Can you work these out from the model? Positions are in its coordinate system, mm. Round coordinates to 2 decimals unless told otherwise and drop trailing zeros. Loops run counter-clockwise (first coordinate to the right, second up) from the corner with the lowest first, then second, coordinate; pieces in that order, holes last. Notation, with made-up numbers: (-27, 62) -> (15, 62) arc R21 ccw to (15, 86) -> close; hole circle Ø7 at (-21.5, 40.25). An arc over 180 degrees is marked (long way). Write each question's results on one line, items separated by ' | '.
from build123d import *

# Parameters (mm, degrees)
SKETCH_1_R          = 27
SKETCH_1_R_2        = 2
EXTRUDE_1_DEPTH     = 5
CUT_EXTRUDE_1_DEPTH = 5
SKETCH_3_R          = 1.6
CUT_EXTRUDE_2_DEPTH = 10


with BuildPart() as part:
    # 草图1 → 凸台-拉伸1 (new body)
    with BuildSketch(Plane(origin=(0, 0, 0), x_dir=(1, 0, 0), z_dir=(0, 1, 0))):
        with Locations(Location((0, 0, 0), (0, 0, 270))):
            Circle(SKETCH_1_R)
        with Locations(Location((0, 0, 0), (0, 0, 270))):
            Circle(SKETCH_1_R_2, mode=Mode.SUBTRACT)
    extrude(amount=EXTRUDE_1_DEPTH)

    # 草图2 → 切除-拉伸1 (cut)
    with BuildSketch(Plane(origin=(0, 5, 0), x_dir=(1, 0, 0), z_dir=(0, 1, 0))):
        Polygon((-3.492969129, -6.05), (3.492969129, -6.05), (6.985938257, 0), (3.492969129, 6.05), (-3.492969129, 6.05), (-6.985938257, 0), align=None)
    extrude(amount=-CUT_EXTRUDE_1_DEPTH, mode=Mode.SUBTRACT)

    # 草图3 → 切除-拉伸2 (cut)
    with BuildSketch(Plane(origin=(0, 5, 0), x_dir=(1, 0, 0), z_dir=(0, 1, 0))):
        with Locations(Location((0, 25, 0), (0, 0, 270))):
            Circle(SKETCH_3_R)
        with Locations(Location((8.550503583, 23.49231552, 0), (0, 0, 270))):
            Circle(SKETCH_3_R)
        with Locations(Location((16.069690242, 19.151111078, 0), (0, 0, 270))):
            Circle(SKETCH_3_R)
        with Locations(Location((21.650635095, 12.5, 0), (0, 0, 270))):
            Circle(SKETCH_3_R)
        with Locations(Location((24.620193825, 4.341204442, 0), (0, 0, 270))):
            Circle(SKETCH_3_R)
        with Locations(Location((24.620193825, -4.341204442, 0), (0, 0, 270))):
            Circle(SKETCH_3_R)
        with Locations(Location((21.650635095, -12.5, 0), (0, 0, 270))):
            Circle(SKETCH_3_R)
        with Locations(Location((16.069690242, -19.151111078, 0), (0, 0, 270))):
            Circle(SKETCH_3_R)
        with Locations(Location((8.550503583, -23.49231552, 0), (0, 0, 270))):
            Circle(SKETCH_3_R)
        with Locations(Location((0, -25, 0), (0, 0, 270))):
            Circle(SKETCH_3_R)
        with Locations(Location((-8.550503583, -23.49231552, 0), (0, 0, 270))):
            Circle(SKETCH_3_R)
        with Locations(Location((-16.069690242, -19.151111078, 0), (0, 0, 270))):
            Circle(SKETCH_3_R)
        with Locations(Location((-21.650635095, -12.5, 0), (0, 0, 270))):
            Circle(SKETCH_3_R)
        with Locations(Location((-24.620193825, -4.341204442, 0), (0, 0, 270))):
            Circle(SKETCH_3_R)
        with Locations(Location((-24.620193825, 4.341204442, 0), (0, 0, 270))):
            Circle(SKETCH_3_R)
        with Locations(Location((-21.650635095, 12.5, 0), (0, 0, 270))):
            Circle(SKETCH_3_R)
        with Locations(Location((-16.069690242, 19.151111078, 0), (0, 0, 270))):
            Circle(SKETCH_3_R)
        with Locations(Location((-8.550503583, 23.49231552, 0), (0, 0, 270))):
            Circle(SKETCH_3_R)
    extrude(amount=-CUT_EXTRUDE_2_DEPTH, mode=Mode.SUBTRACT)


solid = part.part
1. Please list where these lines run through material, in increasing order: line 1 (Z direction, x = -10, y = 0.3); line 2 (Z direction, x = -15.5, y = 0.55); line 3 (X direction, y = 3.4, z = 4.5). Write a range as from..to.
Final values:
line 1: -25.08..-24.17, -22.81..22.81, 24.17..25.08 | line 2: -22.11..-20.65, -17.66..17.66, 20.65..22.11 | line 3: -26.62..-26.21, -23.03..-4.39, 4.39..23.03, 26.21..26.62
2. If we section it at A-A (x = 0): List the corners of the cut face in (y, z) for me.
Final values:
outline: (0, -27) -> (5, -27) -> (5, -26.6) -> (0, -26.6) -> close; (0, -23.4) -> (5, -23.4) -> (5, -6.05) -> (0, -6.05) -> close; (0, 6.05) -> (5, 6.05) -> (5, 23.4) -> (0, 23.4) -> close; (0, 26.6) -> (5, 26.6) -> (5, 27) -> (0, 27) -> close
3. If we section it at B-B (z = 12.5): List the corners of the cut face in (x, y) for me.
Final values:
outline: (-23.93, 0) -> (-23.25, 0) -> (-23.25, 5) -> (-23.93, 5) -> close; (-20.05, 0) -> (20.05, 0) -> (20.05, 5) -> (-20.05, 5) -> close; (23.25, 0) -> (23.93, 0) -> (23.93, 5) -> (23.25, 5) -> close
4. If we section it at C-C (y = 1.25): State how many separate pieces and enclosed holes the cut face has, then the cut area to 3 significant figures.
Final values:
separate pieces: 1 | enclosed holes: 19 | area: 2,020 mm2
5. We'd pull the mould along Z, two halves only. Please class faces 1 (the face through (-23.27, 2.54, 5.2)), 2 (the face through (-26.36, 2.46, -5.85)): pulls with the +Z half, pulls with the -Z half, needs draft (parallel to the pull), parting line crosses it, or undercut.
Final values:
face 1: undercut | face 2: parting line crosses it
6. Will these pins go through, and if not, where does the flat tip stop? pin 1 (1.5 mm diameter, centred on x = -1.5, y = 3, fed in from -Z); pin 2 (1.9 mm diameter, centred on x = -8.55, z = -23.49, fed in from -Y); pin 3 (3 mm diameter, centred on x = 9.5, y = 4, fed in from +Z); pin 4 (2 mm diameter, centred on x = 12, y = 3.5, fed in from -Z).
Final values:
pin 1: z = -26.99 | pin 2: through | pin 3: z = 25.79 | pin 4: z = -24.66
